The drawing under review shows one solid part. Ordinate dimensions are in mm from its lowest x, y, z. A direction names the side the tool comes from. Coordinates: 2 decimals unless noted, no trailing zeros. Write each loop counter-clockwise with the first axis right and the second up, starting at its lowest first coordinate (ties: lowest second). Pieces come first, ordered by that corner, then holes.
1) For P1, Ø2, axis at y = 4.5, z = 28.5, coming from the +X side; P2, Ø8.5, axis at x = 22, z = 10, coming from the +Y side, all flat-tipped, find the tip position at first contact; note any pin that passes through.
2) Add section A-A, the plane x = 22. State the section outline as (y, z) points.
3) Machinability: for the marked faces 1 and 2, which of the approach directions +Z, -Z, +X, -X, +Y, -Y give a long, thin tool a straight path to every point of the face, cutting with its end or side? Answer none if there is none.
4) For line 1 (Y direction, x = 1.15, z = 30); line 2 (Z direction, x = 22, y = 1.95); line 3 (X direction, y = 18, z = 18), list the stretches that pass through material, from the lowest coordinate up.
5) Add section D-D, the plane z = 22.5. State the section outline as (x, y) points, then the cut area to 3 significant figures.
6) Add section C-C, the plane z = 30. State the section outline as (x, y) points, then the cut area to 3 significant figures.
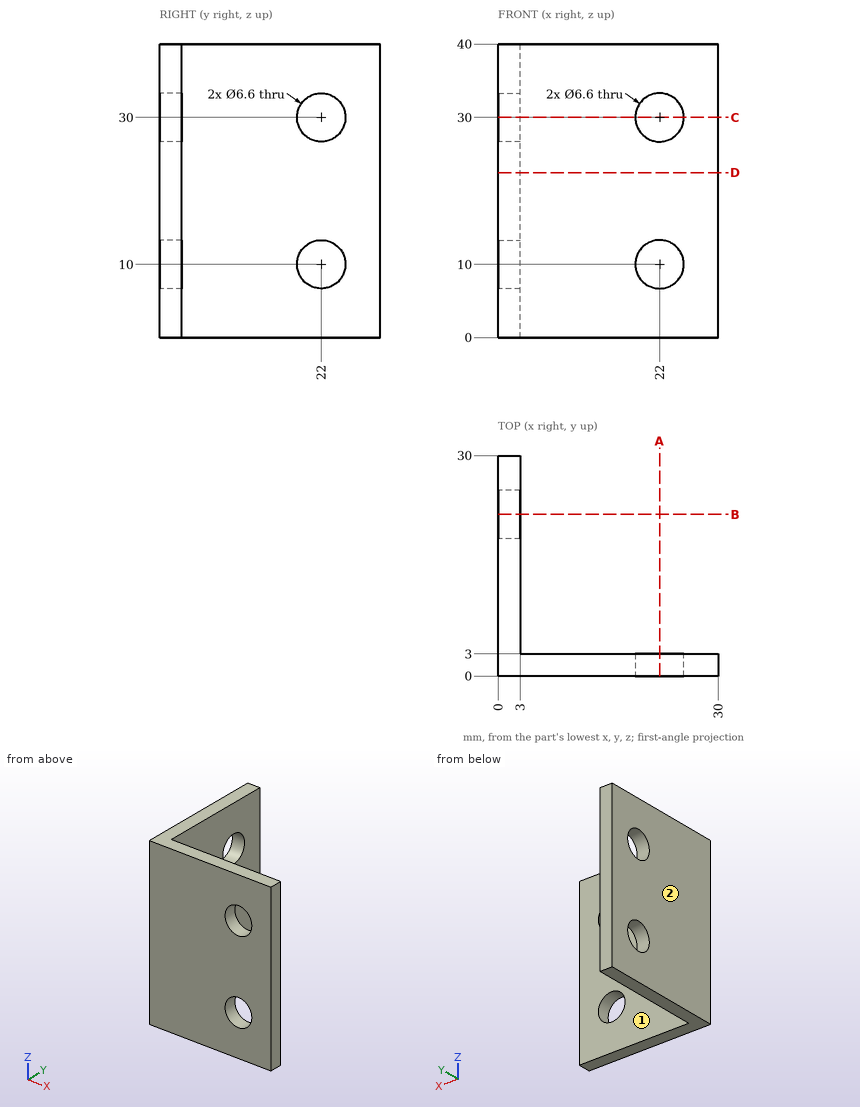
Geometry results:
1. P1: stops at x = 3
1. P2: stops at y = 3
2. outline: (0, 0) - (3, 0) - (3, 6.7) - (0, 6.7) - close; (0, 13.3) - (3, 13.3) - (3, 26.7) - (0, 26.7) - close; (0, 33.3) - (3, 33.3) - (3, 40) - (0, 40) - close
3. face 1: +Z, -Z, +X, +Y
3. face 2: +Z, -Z, -X, +Y, -Y
4. line 1: y = 0 to 18.7, 25.3 to 30
4. line 2: z = 0 to 6.7, 13.3 to 26.7, 33.3 to 40
4. line 3: x = 0 to 3
5. outline: (0, 0) - (30, 0) - (30, 3) - (3, 3) - (3, 30) - (0, 30) - close
5. area: 171 mm2
6. outline: (0, 0) - (18.7, 0) - (18.7, 3) - (3, 3) - (3, 18.7) - (0, 18.7) - close; (0, 25.3) - (3, 25.3) - (3, 30) - (0, 30) - close; (25.3, 0) - (30, 0) - (30, 3) - (25.3, 3) - close
6. area: 131 mm2
